```python
from build123d import *

# Parameters (mm, degrees)
SKETCH1_R           = 4.65
BOSS_EXTRUDE1_DEPTH = 1.4
BOSS_EXTRUDE2_DEPTH = 2.7
SKETCH3_R           = 3.25
BOSS_EXTRUDE3_DEPTH = 1.35
FILLET1_R           = 0.5
CUT_EXTRUDE1_REACH  = 7.45
SKETCH7_R           = 1.925
SKETCH8_R           = 2.75
SKETCH8_R_2         = 1.925
CUT_EXTRUDE2_DEPTH  = 0.1


with BuildPart() as part:
    # Sketch1 → Boss-Extrude1 (new body)
    with BuildSketch(Plane(origin=(0, 0, 0), x_dir=(1, 0, 0), z_dir=(0, 1, 0))):
        Circle(SKETCH1_R)
    extrude(amount=BOSS_EXTRUDE1_DEPTH)

    # Sketch2 → Boss-Extrude2 (add)
    with BuildSketch(Plane(origin=(0, 1.4, 0), x_dir=(1, 0, 0), z_dir=(0, 1, 0))):
        Polygon((0, -3.954849344), (3.425, -1.977424672), (3.425, 1.977424672), (0, 3.954849344), (-3.425, 1.977424672), (-3.425, -1.977424672), align=None)
    extrude(amount=BOSS_EXTRUDE2_DEPTH)

    # Sketch3 → Boss-Extrude3 (add)
    with BuildSketch(Plane(origin=(0, 4.1, 0), x_dir=(1, 0, 0), z_dir=(0, 1, 0))):
        Circle(SKETCH3_R)
    extrude(amount=BOSS_EXTRUDE3_DEPTH)

    # Fillet1
    fillet1_edges = [part.edges().sort_by_distance(p)[0] for p in [
        (-3.25, 5.45, 0),
        (-4.65, 1.4, 0),
    ]]
    fillet(fillet1_edges, radius=FILLET1_R)

    # Sketch7 → Cut-Extrude1 (cut, up to next)
    with BuildSketch(Plane(origin=(0, 5.45, 0), x_dir=(1, 0, 0), z_dir=(0, 1, 0)), mode=Mode.PRIVATE) as cut_extrude1_sk1:
        Circle(SKETCH7_R)
    cut_extrude1_tool1 = extrude(cut_extrude1_sk1.sketch, amount=-CUT_EXTRUDE1_REACH, mode=Mode.PRIVATE) & part.part
    add(cut_extrude1_tool1.solids().sort_by_distance((0, 5.45, 0))[0], mode=Mode.SUBTRACT)

    # Sketch8 → Cut-Extrude2 (cut)
    with BuildSketch(Plane(origin=(0, 5.45, 0), x_dir=(1, 0, 0), z_dir=(0, 1, 0))):
        Circle(SKETCH8_R)
        Circle(SKETCH8_R_2, mode=Mode.SUBTRACT)
    extrude(amount=-CUT_EXTRUDE2_DEPTH, mode=Mode.SUBTRACT)


solid = part.part
```
For this review, take the finished solid that the model builds, in its own axes (mm). A direction names the side the tool comes from. Round coordinates to 2 decimals unless told otherwise and drop trailing zeros. Order: outer loops, then holes, each group sorted by start corner. A loop starts at its lowest first (then second) coordinate and runs counter-clockwise, first axis right, second up.
Q1. We need section D-D, the plane y = 1.15. Give the boundary of the cut face in (x, z) (3 decimals).
Findings below:
outline: circle Ø9.166 at (0, 0); hole circle Ø3.85 at (0, 0)
Q2. Machinability: for faces 5 (the cylindrical face through (-2.579, 4.519, 1.978)), 6 (the flat face through (-1.69, 2.73, -2.98)), 7 (the flat face through (3.425, 3, 0)), which of the approach directions +Z, -Z, +X, -X, +Y, -Y give a long, thin tool a straight path to every point of the face, cutting with its end or side? Answer none if there is none.
Findings below:
face 5: +Y
face 6: -Z, -X, +Y
face 7: +Z, -Z, +X, +Y
Q3. Wall thickness on line 1 (X direction, y = 2.4, z = 0) (3 decimals); line 2 (Z direction, x = 0, y = 4.4) (3 decimals); line 3 (Y direction, x = -3, z = 1.75): over which ranges is each line inside the solid? List them lowest first.
Findings below:
line 1: x = -3.425 to -1.925, 1.925 to 3.425
line 2: z = -3.25 to -1.925, 1.925 to 3.25
line 3: y = 0 to 4.1
Q4. We need section B-B, the plane y = 3.5. Give the boundary of the cut face in (x, z) (3 decimals), plus the area to 3 significant figures.
Findings below:
outline: (-3.425, -1.977) - (0, -3.955) - (3.425, -1.977) - (3.425, 1.977) - (0, 3.955) - (-3.425, 1.977) - close; hole circle Ø3.85 at (0, 0)
area: 29.0 mm2
Q5. Insertion check: P1, Ø2, axis at y = 3, z = 0, coming from the -X side (3 decimals); P2, Ø0.8, axis at y = 2.5, z = -0.5, coming from the +X side (3 decimals); P3, Ø3.5, axis at x = -1.5, z = -0.5, coming from the +Y side; P4, Ø1, axis at x = 2, y = 2, coming from the +Z side. Each pin has a flat end and moves straight along its axis. Give the tip position at first contact, or say it passes through.
Findings below:
P1: stops at x = -3.425
P2: stops at x = 3.425
P3: stops at y = 5.45
P4: stops at z = 3.09
Q6. We need section C-C, the plane y = 4.4. Give the boundary of the cut face in (x, z) (3 decimals), plus the area to 3 significant figures.
Findings below:
outline: circle Ø6.5 at (0, 0); hole circle Ø3.85 at (0, 0)
area: 21.5 mm2
Q7. Mouldability with a two-part tool opening along X and no side actions: class faces 1 (the flat face through (-3.425, 3, 0)), 2 (the cylindrical face through (2.5, 0.44, -3.92)), 3 (the flat face through (1, 5.35, -2)), 4 (the flat face through (1.69, 2.73, 2.98)) as pulls with the +X half, pulls with the -X half, needs draft (parallel to the pull), parting line crosses it, or undercut.
Findings below:
face 1: pulls with the -X half
face 2: parting line crosses it
face 3: undercut
face 4: pulls with the +X half
Q8. We need section A-A, the plane z = 0. Give the boundary of the cut face in (x, y) (3 decimals).
Findings below:
outline: (-4.65, 0) - (-1.925, 0) - (-1.925, 5.35) - (-2.75, 5.35) - (-2.75, 5.45) arc R0.5 ccw to (-3.25, 4.95) - (-3.25, 4.1) - (-3.425, 4.1) - (-3.425, 1.4) - (-4.15, 1.4) arc R0.5 ccw to (-4.65, 0.9) - close; (1.925, 0) - (4.65, 0) - (4.65, 0.9) arc R0.5 ccw to (4.15, 1.4) - (3.425, 1.4) - (3.425, 4.1) - (3.25, 4.1) - (3.25, 4.95) arc R0.5 ccw to (2.75, 5.45) - (2.75, 5.35) - (1.925, 5.35) - close
